```python
from build123d import *

# Parameters (mm, degrees)
SKETCH1_R           = 4
SKETCH1_R_2         = 2.5
BOSS_EXTRUDE1_DEPTH = 3


with BuildPart() as part:
    # Sketch1 → Boss-Extrude1 (new body)
    with BuildSketch(Plane(origin=(0, 0, 0), x_dir=(1, 0, 0), z_dir=(0, 1, 0))):
        with BuildLine():
            Line((-56, 21.5), (-61.341258546, 21.5))
            ThreePointArc((-61.341258546, 21.5), (-45.961940777, 45.961940777), (-21.5, 61.341258546))
            Line((-21.5, 61.341258546), (-21.5, 56))
            ThreePointArc((-21.5, 56), (0, 34.5), (21.5, 56))
            Line((21.5, 56), (21.5, 61.341258546))
            ThreePointArc((21.5, 61.341258546), (45.961940777, 45.961940777), (61.341258546, 21.5))
            Line((61.341258546, 21.5), (56, 21.5))
            ThreePointArc((56, 21.5), (34.5, 0), (56, -21.5))
            Line((56, -21.5), (61.341258546, -21.5))
            ThreePointArc((61.341258546, -21.5), (45.961940777, -45.961940777), (21.5, -61.341258546))
            Line((21.5, -61.341258546), (21.5, -56))
            ThreePointArc((21.5, -56), (0, -34.5), (-21.5, -56))
            Line((-21.5, -56), (-21.5, -61.341258546))
            ThreePointArc((-21.5, -61.341258546), (-45.961940777, -45.961940777), (-61.341258546, -21.5))
            Line((-61.341258546, -21.5), (-56, -21.5))
            ThreePointArc((-56, -21.5), (-34.5, 0), (-56, 21.5))
        make_face()
        with Locations(Location((0, 0, 0), (0, 0, 270))):
            Circle(SKETCH1_R, mode=Mode.SUBTRACT)
        with Locations(Location((-31.819805153, 31.819805153, 0), (0, 0, 270))):
            Circle(SKETCH1_R_2, mode=Mode.SUBTRACT)
        with Locations(Location((31.819805153, 31.819805153, 0), (0, 0, 270))):
            Circle(SKETCH1_R_2, mode=Mode.SUBTRACT)
        with Locations(Location((31.819805153, -31.819805153, 0), (0, 0, 270))):
            Circle(SKETCH1_R_2, mode=Mode.SUBTRACT)
        with Locations(Location((-31.819805153, -31.819805153, 0), (0, 0, 270))):
            Circle(SKETCH1_R_2, mode=Mode.SUBTRACT)
    extrude(amount=BOSS_EXTRUDE1_DEPTH)


solid = part.part
```
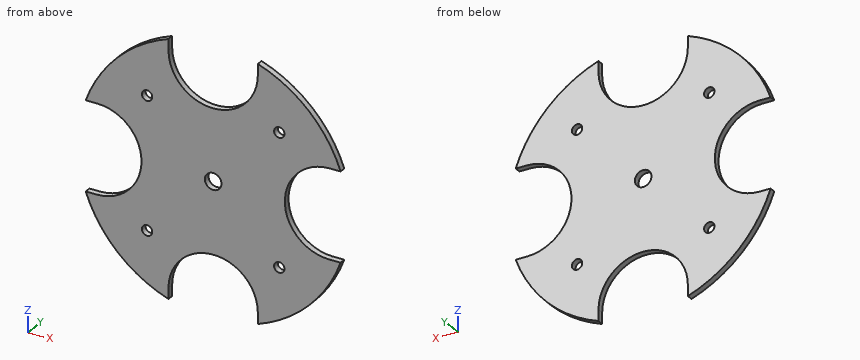
Design review of the part built by this model. Coordinates are the model's own, in mm. Coordinates: 2 decimals unless noted, no trailing zeros. Order: outer loops, then holes, each group sorted by start corner. A loop starts at its lowest first (then second) coordinate and runs counter-clockwise, first axis right, second up.
1) Take a section at D-D, the plane x = 26.5. Give the boundary of the cut face in (y, z).
2) Wall thickness on line 1 along Z through (x, y) = (-34, 0.45); line 2 along X through (y, z) = (0.35, -31.5); line 3 along X through (y, z) = (1.8, -31): over which ranges is each line inside the solid? List them lowest first.
3) Clearance check with flat-ended pins moving along their axes: pin 1 (0.9 mm diameter, centred on y = 2, z = -58, fed in from +X); pin 2 (1.5 mm diameter, centred on y = 2, z = -59, fed in from -X); pin 3 (6 mm diameter, centred on x = 28.5, z = -24, fed in from -Y); pin 4 (0.9 mm diameter, centred on x = 58.5, y = 2, fed in from +Z). State where each tip first meets the part, or that it passes through.
4) Take a section at B-B, the plane z = 36.5. Give the boundary of the cut face in (x, y).
5) Take a section at A-A, the plane x = 0. Give the boundary of the cut face in (y, z), and give its area (3 significant figures).
6) Take a section at C-C, the plane y = 2.45. Give the boundary of the cut face in (x, z), and give its area (3 significant figures).
Returned:
1. outline: (0, -59.35) - (3, -59.35) - (3, 59.35) - (0, 59.35) - close
2. line 1: z = -55.4 to -33.04, -30.6 to 30.6, 33.04 to 55.4
2. line 2: x = -56.86 to -34.3, -29.34 to 29.34, 34.3 to 56.86
2. line 3: x = -57.13 to -34.18, -29.46 to 29.46, 34.18 to 57.13
3. pin 1: stops at x = 30.22
3. pin 2: stops at x = -28.84
3. pin 3: stops at y = 0
3. pin 4: stops at z = 29.24
4. outline: (-53.78, 0) - (-9.06, 0) - (-9.06, 3) - (-53.78, 3) - close; (9.06, 0) - (53.78, 0) - (53.78, 3) - (9.06, 3) - close
5. outline: (0, -34.5) - (3, -34.5) - (3, -4) - (0, -4) - close; (0, 4) - (3, 4) - (3, 34.5) - (0, 34.5) - close
5. area: 183 mm2
6. outline: (-61.34, -21.5) arc R65 ccw to (-21.5, -61.34) - (-21.5, -56) arc R21.5 cw to (21.5, -56) - (21.5, -61.34) arc R65 ccw to (61.34, -21.5) - (56, -21.5) arc R21.5 cw to (56, 21.5) - (61.34, 21.5) arc R65 ccw to (21.5, 61.34) - (21.5, 56) arc R21.5 cw to (-21.5, 56) - (-21.5, 61.34) arc R65 ccw to (-61.34, 21.5) - (-56, 21.5) arc R21.5 cw to (-56, -21.5) - close; hole circle Ø5 at (-31.82, -31.82); hole circle Ø5 at (-31.82, 31.82); hole circle Ø8 at (0, 0); hole circle Ø5 at (31.82, -31.82); hole circle Ø5 at (31.82, 31.82)
6. area: 8,900 mm2
